The listing builds one solid part. Answer for the finished solid, in the listing's coordinates (mm). A direction names the side the tool comes from. Coordinates: 2 decimals unless noted, no trailing zeros. Loops run counter-clockwise (first coordinate to the right, second up) from the corner with the lowest first, then second, coordinate; pieces in that order, holes last. Notation, with made-up numbers: M 71.25,41.5 L 89.25,41.5 A21 cw 89.25,54.5 Z; hole C 26.25,73 d1. An arc over 180 degrees is marked long. Answer in a Markdown table with one row per item. Add a question column.
from build123d import *

# Parameters (mm, degrees)
F0_R     = 10
F1_DEPTH = 1
F3_R     = 8
F4_DEPTH = 4
F5_R     = 6
F6_DEPTH = 4
F7_W     = 17.3227433115
F7_H     = 1.3524350361
F8_DEPTH = 25
F9_R     = 0.5


# Not quite as in the source:
# - a fillet or chamfer that OpenCascade refuses, or shapes differently, is made with other operations: its cross-section is extruded or revolved along the edge and cut away or added


with BuildPart() as f1:
    # F0 (on Top) → F1 (new body)
    with BuildSketch(Plane.XY):
        Circle(F0_R)
    extrude(amount=F1_DEPTH)

    # F2: fillet of radius 2 on 1 edges, made by hand

    # F2_s1 → F2_t2 (revolve, cut)
    with BuildSketch(Plane.XZ):
        with BuildLine():
            ThreePointArc((10, 1), (9.2679491924, 0.2679491924), (8.2679491924, 0))
            Line((8.2679491924, 0), (10, 0))
            Line((10, 0), (10, 1))
        make_face()
    revolve(axis=Axis((0, 0, 0), (0, 0, 1)), mode=Mode.SUBTRACT)

    # F3 (on face) → F4 (join)
    with BuildSketch(Plane.XY.offset(1)):
        Circle(F3_R)
    extrude(amount=F4_DEPTH)

    # F5 (on face) → F6 (cut)
    with BuildSketch(Plane.XY.offset(5)):
        Circle(F5_R)
    extrude(amount=-F6_DEPTH, mode=Mode.SUBTRACT)

    # F7 (on face) → F8 (cut)
    with BuildSketch(Plane.XY.offset(1)):
        with Locations((-0.0975718722, 0.0086750078)):
            Rectangle(F7_W, F7_H)
    extrude(amount=F8_DEPTH, mode=Mode.SUBTRACT)

    # F9
    f9_edges = [f1.edges().sort_by_distance(p)[0] for p in [
        (0, 8, 5),
        (0, -8, 5),
    ]]
    fillet(f9_edges, radius=F9_R)


solid = f1.part
(1) Straight lines are drawn through the part: line 1 (Z direction, x = 1, y = 3.5); line 2 (X direction, y = 0.75, z = 4.5); line 3 (Y direction, x = -4, z = 4.5). For each, find the intervals that lie inside material, in ascending order.
(2) A cutting plane is placed at B-B (z = 0.6). Give the vertices of the cut face in (x, y), plus the area to 3 significant figures.
(3) A cutting plane is placed at A-A (z = 2.2). Give the vertices of the cut face in (x, y), plus the area to 3 significant figures.
(4) For faces 1 (the face through (0, 8, 3)), 2 (the face through (0.52, 6.13, 5)), 3 (the face through (-7, 0.685, 3)), determine the directions among +Z, -Z, +X, -X, +Y, -Y from which every point of the face is accessible in a straight line to the end or side of a thin tool.
(5) Each of these flat-tipped pins is pushed along its axis until it touches: pin 1 (1.6 mm diameter, centred on x = -7, z = 3, fed in from -Y); pin 2 (0.6 mm diameter, centred on x = -7, z = 2.5, fed in from +Y); pin 3 (0.6 mm diameter, centred on x = 7, z = 2.5, fed in from -Y). Where does it stop, or does it pass through?
(6) The mould has two halves that part along X. Classify faces 4 (the face through (0, -6, 3)), 5 (the face through (7, 0.685, 3)), 6 (the face through (0, -8, 3)), 7 (the face through (0, 6, 3)): released by +X, released by -X, zero draft, split by the parting line, or undercut.
Solved:
| question | item | result |
|---|---|---|
| 1 | line 1 | z = 0 to 1 |
| 1 | line 2 | x = -7.96 to -5.95, 5.95 to 7.96 |
| 1 | line 3 | y = -6.93 to -4.47, 4.47 to 6.93 |
| 2 | outline | C 0,0 d19.39 |
| 2 | area | 295 mm² |
| 3 | outline | M -7.97,-0.67 A8 ccw 7.97,-0.67 L 5.96,-0.67 A6 cw -5.96,-0.67 Z; M -7.97,0.68 L -5.96,0.68 A6 cw 5.96,0.68 L 7.97,0.68 A8 ccw Z |
| 3 | area | 82.5 mm² |
| 4 | face 1 | +Z, +Y |
| 4 | face 2 | +Z, +X, -X, +Y, -Y |
| 4 | face 3 | +Z, +X, -X |
| 5 | pin 1 | stops at y = -5.06 |
| 5 | pin 2 | stops at y = 4.37 |
| 5 | pin 3 | stops at y = -4.37 |
| 6 | face 4 | undercut |
| 6 | face 5 | zero draft |
| 6 | face 6 | split by the parting line |
| 6 | face 7 | undercut |
